Here's how the part is built. I have some questions about the finished solid (model axes, mm). Coordinates: 2 decimals unless noted, no trailing zeros. Loops run counter-clockwise (first coordinate to the right, second up) from the corner with the lowest first, then second, coordinate; pieces in that order, holes last. Notation, with made-up numbers: M -14,-12.5 L 4,-12.5 A25 cw 4,2.5 Z; hole C -23,-6 d2. An arc over 180 degrees is marked long. Use CSV: the item, a comma, the result in double quotes. Start each with the question number.
Q1. If we section it at C-C (x = -55.5): Please give me the cut outline in (y, z).
Q2. For pin 1 Ø2.5 at (y, z) = (28.5, 2) entering from -X; pin 2 Ø3.5 at (y, z) = (-32.5, 2) entering from +X; pin 3 Ø0.6 at (x, y) = (-78.5, -57) entering from +Z; pin 4 Ø2 at (x, y) = (-78.5, 58) entering from -Z, each with a flat end and sliding along its axis, tell me the tip position at first contact or that it passes through.
Q3. If we section it at B-B (y = 44): Please give me the cut outline in (x, z).
Q4. Please list where these lines run through material, in increasing order: probe 1 along X at (y, z) = (58, -0.8); probe 2 along X at (y, z) = (-41.25, 2.7) (3 decimals); probe 3 along Y at (x, z) = (-78.5, -1). Write a range as [from, to].
Q5. If we section it at A-A (x = -19.5): Please give me the cut outline in (y, z).
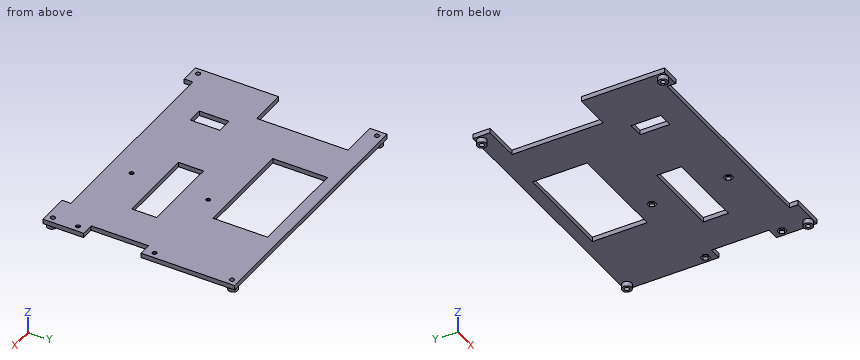
from build123d import *

# Parameters (mm, degrees)
CROQUIS9_W              = 165
CROQUIS9_H              = 122.5
CROQUIS9_R              = 1.5
SALIENTE_EXTRUIR7_DEPTH = 3
CROQUIS10_R             = 3
CROQUIS10_R_2           = 1.5
SALIENTE_EXTRUIR4_DEPTH = 3
CROQUIS13_R             = 1.375
CORTAR_EXTRUIR6_DEPTH   = 7
CORTAR_EXTRUIR9_DEPTH   = 2
CROQUIS19_W             = 23.751706854
CROQUIS19_H             = 58.322995046
CORTAR_EXTRUIR11_DEPTH  = 7
CROQUIS20_W             = 8.074798139
CROQUIS20_H             = 36.716786424
CORTAR_EXTRUIR12_DEPTH  = 7
CROQUIS21_W             = 132.215541909
CROQUIS21_H             = 5.552865293
CORTAR_EXTRUIR13_DEPTH  = 7
CROQUIS22_W             = 64.97984938
CROQUIS22_H             = 34.980531845
CORTAR_EXTRUIR14_DEPTH  = 10
CROQUIS23_W             = 9.785151637
CROQUIS23_H             = 18.811760375
CORTAR_EXTRUIR15_DEPTH  = 7
CROQUIS24_W             = 50.724588702
CROQUIS24_H             = 15.98003992
CORTAR_EXTRUIR16_DEPTH  = 10


with BuildPart() as part:
    # Croquis9 → Saliente-Extruir7 (new body)
    with BuildSketch(Plane(origin=(0, -39.711212197, 0), x_dir=(-1, 0, 0), z_dir=(0, 0, 1))):
        with Locations((0, -39.711212197)):
            Rectangle(CROQUIS9_W, CROQUIS9_H)
        with Locations((-78.5, 17.538787803)):
            Circle(CROQUIS9_R, mode=Mode.SUBTRACT)
        with Locations((78.5, 17.538787803)):
            Circle(CROQUIS9_R, mode=Mode.SUBTRACT)
        with Locations((-78.5, -96.961212197)):
            Circle(CROQUIS9_R, mode=Mode.SUBTRACT)
        with Locations((78.5, -96.961212197)):
            Circle(CROQUIS9_R, mode=Mode.SUBTRACT)
    extrude(amount=SALIENTE_EXTRUIR7_DEPTH)

    # Croquis10 → Saliente-Extruir4 (add)
    with BuildSketch(Plane(origin=(0, -39.711212197, 0), x_dir=(1, 0, 0), z_dir=(0, 0, -1))):
        with Locations((-78.5, 18.288787803)):
            Circle(CROQUIS10_R)
        with Locations((-78.5, 18.288787803)):
            Circle(CROQUIS10_R_2, mode=Mode.SUBTRACT)
        with Locations((78.5, 18.288787803)):
            Circle(CROQUIS10_R)
        with Locations((78.5, 18.288787803)):
            Circle(CROQUIS10_R_2, mode=Mode.SUBTRACT)
        with Locations((78.5, -97.711212197)):
            Circle(CROQUIS10_R)
        with Locations((78.5, -97.711212197)):
            Circle(CROQUIS10_R_2, mode=Mode.SUBTRACT)
        with Locations((-78.5, -97.711212197)):
            Circle(CROQUIS10_R)
        with Locations((-78.5, -97.711212197)):
            Circle(CROQUIS10_R_2, mode=Mode.SUBTRACT)
    extrude(amount=SALIENTE_EXTRUIR4_DEPTH)

    # Croquis13 → Cortar-Extruir6 (cut, through all)
    with BuildSketch(Plane(origin=(0, -58.652466741, 3), x_dir=(1, 0, 0), z_dir=(0, 0, -1))):
        with Locations((20.5, -17.402466741)):
            Circle(CROQUIS13_R)
        with Locations((78.5, -17.402466741)):
            Circle(CROQUIS13_R)
        with Locations((20.5, -66.402466741)):
            Circle(CROQUIS13_R)
        with Locations((78.5, -66.402466741)):
            Circle(CROQUIS13_R)
    extrude(amount=CORTAR_EXTRUIR6_DEPTH, mode=Mode.SUBTRACT)

    # Croquis17 → Cortar-Extruir9 (cut)
    with BuildSketch(Plane(origin=(0, -39.711212197, 0), x_dir=(1, 0, 0), z_dir=(0, 0, -1))):
        Polygon((23.340563324, 1.538787803), (21.920281662, 3.998787803), (19.079718338, 3.998787803), (17.659436676, 1.538787803), (19.079718338, -0.921212197), (21.920281662, -0.921212197), align=None)
        Polygon((81.340563324, 1.538787803), (79.920281662, 3.998787803), (77.079718338, 3.998787803), (75.659436676, 1.538787803), (77.079718338, -0.921212197), (79.920281662, -0.921212197), align=None)
        Polygon((81.340563324, -47.461212197), (79.920281662, -45.001212197), (77.079718338, -45.001212197), (75.659436676, -47.461212197), (77.079718338, -49.921212197), (79.920281662, -49.921212197), align=None)
        Polygon((23.340563324, -47.461212197), (21.920281662, -45.001212197), (19.079718338, -45.001212197), (17.659436676, -47.461212197), (19.079718338, -49.921212197), (21.920281662, -49.921212197), align=None)
    extrude(amount=-CORTAR_EXTRUIR9_DEPTH, mode=Mode.SUBTRACT)

    # Croquis19 → Cortar-Extruir11 (cut, through all)
    with BuildSketch(Plane.XY.offset(3)):
        with Locations((-70.624146573, 21.159042343)):
            Rectangle(CROQUIS19_W, CROQUIS19_H)
    extrude(amount=-CORTAR_EXTRUIR11_DEPTH, mode=Mode.SUBTRACT)

    # Croquis20 → Cortar-Extruir12 (cut, through all)
    with BuildSketch(Plane.XY.offset(3)):
        with Locations((78.462600931, -16.844106748)):
            Rectangle(CROQUIS20_W, CROQUIS20_H)
    extrude(amount=-CORTAR_EXTRUIR12_DEPTH, mode=Mode.SUBTRACT)

    # Croquis21 → Cortar-Extruir13 (cut, through all)
    with BuildSketch(Plane.XY.offset(3)):
        with Locations((-4.222973471, -58.473567354)):
            Rectangle(CROQUIS21_W, CROQUIS21_H)
    extrude(amount=-CORTAR_EXTRUIR13_DEPTH, mode=Mode.SUBTRACT)

    # Croquis22 → Cortar-Extruir14 (cut)
    with BuildSketch(Plane.XY.offset(3)):
        with Locations((1.632848722, 36.266393101)):
            Rectangle(CROQUIS22_W, CROQUIS22_H)
    extrude(amount=-CORTAR_EXTRUIR14_DEPTH, mode=Mode.SUBTRACT)

    # Croquis23 → Cortar-Extruir15 (cut, through all)
    with BuildSketch(Plane.XY.offset(3)):
        with Locations((-43.761194105, -29.321605041)):
            Rectangle(CROQUIS23_W, CROQUIS23_H)
    extrude(amount=-CORTAR_EXTRUIR15_DEPTH, mode=Mode.SUBTRACT)

    # Croquis24 → Cortar-Extruir16 (cut)
    with BuildSketch(Plane(origin=(0, 0, 0), x_dir=(-1, 0, 0), z_dir=(0, 0, -1))):
        with Locations((-23.977071959, -16.156592187)):
            Rectangle(CROQUIS24_W, CROQUIS24_H)
    extrude(amount=-CORTAR_EXTRUIR16_DEPTH, mode=Mode.SUBTRACT)


solid = part.part
Results below:
1,outline,"M -55.7,0 L 61.25,0 L 61.25,3 L -55.7,3 Z"
2,pin 1,"x = -58.75"
2,pin 2,"x = 74.43"
2,pin 3,"through"
2,pin 4,"z = 0"
3,outline,"M -58.75,0 L -30.86,0 L -30.86,3 L -58.75,3 Z; M 34.12,0 L 82.5,0 L 82.5,3 L 34.12,3 Z"
4,probe 1,"[-81.5, -80], [-77, -75.5], [75.5, 77], [80, 81.5]"
4,probe 2,"[-82.5, 19.125], [21.875, 77.125], [79.875, 82.5]"
4,probe 3,"[-61, -59.5], [-56.5, -55], [55, 56.5], [59.5, 61]"
5,outline,"M -55.7,0 L 18.78,0 L 18.78,3 L -55.7,3 Z; M 53.76,0 L 61.25,0 L 61.25,3 L 53.76,3 Z"
